from build123d import *

# Parameters (mm, degrees)
CROQUIS1_R              = 12.5
SALIENTE_EXTRUIR1_DEPTH = 600
CROQUIS2_R              = 15
SALIENTE_EXTRUIR2_DEPTH = 8


with BuildPart() as part:
    # Croquis1 → Saliente-Extruir1 (new body)
    with BuildSketch(Plane.XY):
        Circle(CROQUIS1_R)
    extrude(amount=-SALIENTE_EXTRUIR1_DEPTH)

    # Croquis2 → Saliente-Extruir2 (add)
    with BuildSketch(Plane.XY):
        Circle(CROQUIS2_R)
    saliente_extruir2 = extrude(amount=SALIENTE_EXTRUIR2_DEPTH)

    # Simetría1: Saliente-Extruir2 across plane
    add(saliente_extruir2.mirror(Plane.XY.offset(-300)))


solid = part.part
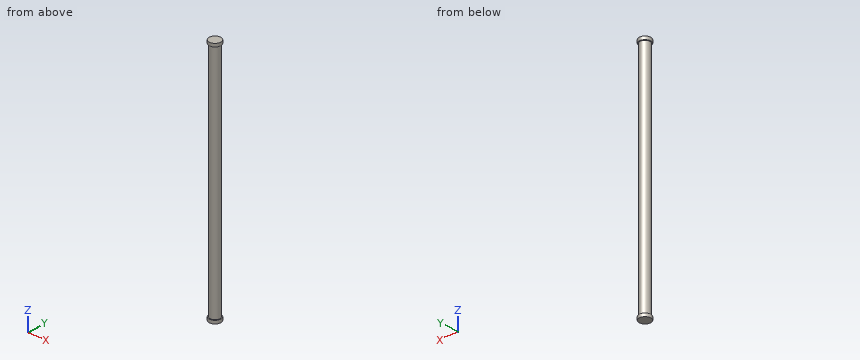
Could you check a few things on this model? Use its own coordinates, in mm. Give positions to 0.01 mm unless a question says otherwise; leave off trailing zeros. Write each loop counter-clockwise with the first axis right and the second up, starting at its lowest first coordinate (ties: lowest second). Pieces come first, ordered by that corner, then holes. Notation, with made-up numbers: (-23, -15.5) - (1, -15.5) arc R20 ccw to (1, -11.5) - close; hole circle Ø2 at (19, -29). An arc over 180 degrees is marked (long way). Use CSV: the item, a comma, the result in double quotes. Start each with the question number.
Item 1: If I drill on line 1 along Z through (x, y) = (6.5, 12); line 2 along X through (y, z) = (0.5, -505.5); line 3 along Y through (x, z) = (0.75, -345), over which ranges is the centre line in solid material (lowest first)?
Item 2: I want a section at C-C, the plane z = -444.5. Please give me the cut outline in (x, y), then the cut area to 3 significant figures.
Item 3: I'm going to push flat-ended pins straight in: pin 1 (1 mm diameter, centred on y = -10.5, z = -240.5, fed in from +X); pin 2 (4 mm diameter, centred on x = -11, z = -264, fed in from -Y); pin 3 (1 mm diameter, centred on y = 1, z = -136.5, fed in from +X). Where does each tip first touch, or does it pass through?
Item 4: I want a section at A-A, the plane y = 0. Please give me the cut outline in (x, z).
Findings:
1,line 1,"z = -608 to -600, 0 to 8"
1,line 2,"x = -12.49 to 12.49"
1,line 3,"y = -12.48 to 12.48"
2,outline,"circle Ø25 at (0, 0)"
2,area,"491 mm2"
3,pin 1,"stops at x = 7.5"
3,pin 2,"stops at y = -8.67"
3,pin 3,"stops at x = 12.49"
4,outline,"(-15, -608) - (15, -608) - (15, -600) - (12.5, -600) - (12.5, 0) - (15, 0) - (15, 8) - (-15, 8) - (-15, 0) - (-12.5, 0) - (-12.5, -600) - (-15, -600) - close"
